```python
from build123d import *


with BuildPart() as part:
    # Schizzo1 → Rivoluzione1 (revolve)
    with BuildSketch(Plane(origin=(0, 0, 0), x_dir=(-1, 0, 0), z_dir=(0, 0, 1)), mode=Mode.PRIVATE) as rivoluzione1_sk:
        with BuildLine():
            Line((-554.694489339, -544.755446129), (-379.995479902, -588.120248731))
            ThreePointArc((-379.995479902, -588.120248731), (-363.473567073, -591.36496946), (-346.694145738, -592.762408471))
            Line((-346.694145738, -592.762408471), (-188.558838555, -568.406205519))
            Line((-188.558838555, -568.406205519), (-5.145007861, -549.45847961))
            Line((-5.145007861, -549.45847961), (4.842484317, -549.45847961))
            Line((4.842484317, -549.45847961), (4.842484317, -549.55847961))
            Line((4.842484317, -549.55847961), (-5.139856275, -549.55847961))
            Line((-5.139856275, -549.55847961), (-188.546081358, -568.505419815))
            Line((-188.546081358, -568.505419815), (-346.687865577, -592.862620368))
            ThreePointArc((-346.687865577, -592.862620368), (-363.482742045, -591.464657333), (-380.01986383, -588.217230765))
            Line((-380.01986383, -588.217230765), (-554.718580803, -544.852500759))
            Line((-554.718580803, -544.852500759), (-554.694489339, -544.755446129))
        make_face()
    revolve(rivoluzione1_sk.sketch.rotate(Axis((-4.842484317, 549.239933768, 0), (0, 1, 0)), 90), axis=Axis((-4.842484317, 549.239933768, 0), (0, 1, 0)))


solid = part.part
```
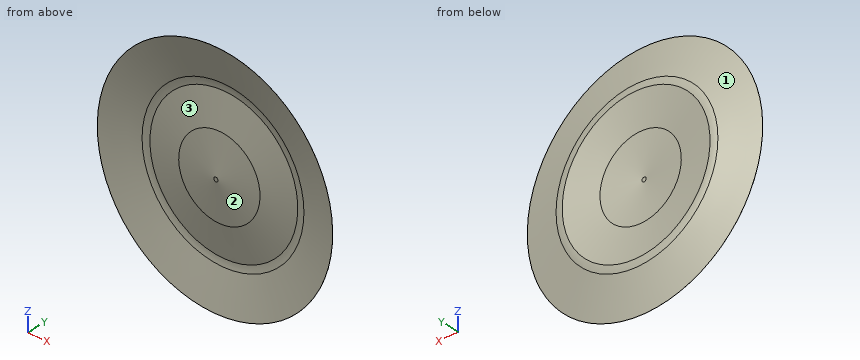
The model under review builds one solid part; all positions refer to its coordinate system, in mm. Face numbers are marked on the shaded views. Give positions to 0.01 mm unless a question says otherwise; leave off trailing zeros. Loops run counter-clockwise (first coordinate to the right, second up) from the corner with the lowest first, then second, coordinate; pieces in that order, holes last. Notation, with made-up numbers: (70, 61) -> (92, 61) arc R26 ccw to (92, 99) -> close; hole circle Ø11 at (66.5, 6). An arc over 180 degrees is marked (long way). Use CSV: the item, a comma, the result in double quotes.
1. For P1, Ø8, axis at x = 218, z = -364, coming from the +Y side; P2, Ø22, axis at x = -4.5, z = -1, coming from the -Y side; P3, Ø10, axis at x = -395, z = -6.5, coming from the -Y side, all flat-tipped, find the tip position at first contact; note any pin that passes through.
Result:
P1,"stops at y = 578.8"
P2,"stops at y = 549.46"
P3,"stops at y = 585.55"
2. Consider section A-A, the plane y = 557.5. Write out the cut boundary in (x, z), then the cut area to 3 significant figures.
Result:
outline,"circle Ø1017.22 at (-4.84, 0); circle Ø175.66 at (-4.84, 0); hole circle Ø1016.39 at (-4.84, 0); hole circle Ø173.71 at (-4.84, 0)"
area,"1,860 mm²"
3. The part is to be moulded in two halves that separate along Z. For the marked faces 1, 2 and 3, say which applies: +Z half, -Z half, draft (parallel to the pull), parting line (faces both ways), or undercut.
Result:
face 1,"parting line"
face 2,"undercut"
face 3,"undercut"
